```python
from build123d import *

# Parameters (mm, degrees)
SKETCH_1_R             = 10.5
EXTRUDE_1_DEPTH        = 4
SKETCH_4_R             = 2.1
CUT_EXTRUDE_1346_DEPTH = 150.081575092


with BuildPart() as part:
    # 草图1 → 凸台-拉伸1 (new body)
    with BuildSketch(Plane(origin=(0, 0, 0), x_dir=(1, 0, 0), z_dir=(0, 1, 0))):
        with BuildLine():
            Line((0, 0), (60, 0))
            Line((60, 0), (60, 10))
            Line((60, 10), (55.411884484, 19.839245477))
            ThreePointArc((55.411884484, 19.839245477), (55.227167567, 21.861337052), (56.372632354, 23.537906496))
            ThreePointArc((56.372632354, 23.537906496), (70.783850417, 79.017821778), (19.020417199, 103.639990393))
            ThreePointArc((19.020417199, 103.639990393), (16.99979992, 103.840191523), (15.569521651, 105.281468301))
            Line((15.569521651, 105.281468301), (9.668235965, 117.936816295))
            ThreePointArc((9.668235965, 117.936816295), (-13.775496492, 127.647528231), (-25.492512153, 105.139350566))
            Line((-25.492512153, 105.139350566), (0, 10))
            Line((0, 10), (0, 0))
        make_face()
        with Locations(Location((-7.352321507, 110, 0), (0, 0, 270))):
            Circle(SKETCH_1_R, mode=Mode.SUBTRACT)
        with BuildLine():
            Line((26.5, 20.5), (31.5, 20.5))
            ThreePointArc((31.5, 20.5), (32.5, 19.5), (31.5, 18.5))
            Line((31.5, 18.5), (26.5, 18.5))
            ThreePointArc((26.5, 18.5), (25.5, 19.5), (26.5, 20.5))
        make_face(mode=Mode.SUBTRACT)
        with BuildLine():
            Line((-0.975772037, 35.443910191), (2.27680142, 31.646441837))
            ThreePointArc((2.27680142, 31.646441837), (2.167822441, 30.236433474), (0.757814079, 30.345412454))
            Line((0.757814079, 30.345412454), (-2.494759379, 34.142880808))
            ThreePointArc((-2.494759379, 34.142880808), (-2.3857804, 35.552889171), (-0.975772037, 35.443910191))
        make_face(mode=Mode.SUBTRACT)
        with BuildLine():
            Line((60.975772037, 35.443910191), (57.72319858, 31.646441837))
            ThreePointArc((57.72319858, 31.646441837), (57.832177559, 30.236433474), (59.242185921, 30.345412454))
            Line((59.242185921, 30.345412454), (62.494759379, 34.142880808))
            ThreePointArc((62.494759379, 34.142880808), (62.3857804, 35.552889171), (60.975772037, 35.443910191))
        make_face(mode=Mode.SUBTRACT)
    extrude(amount=EXTRUDE_1_DEPTH)

    # 草图4 → Cut-Extrude 1346 (cut, through all)
    with BuildSketch(Plane.XZ):
        with Locations(Location((37, -5, 0), (0, 0, 270))):
            Circle(SKETCH_4_R)
        with Locations(Location((51, -5, 0), (0, 0, 270))):
            Circle(SKETCH_4_R)
        with Locations(Location((9, -5, 0), (0, 0, 90))):
            Circle(SKETCH_4_R)
        with Locations(Location((23, -5, 0), (0, 0, 90))):
            Circle(SKETCH_4_R)
    extrude(amount=-CUT_EXTRUDE_1346_DEPTH, mode=Mode.SUBTRACT)


solid = part.part
```
Model file for the job. Use its own axes, mm. A direction names the side the tool comes from. Give positions to 0.01 mm unless a question says otherwise; leave off trailing zeros. Write each loop counter-clockwise with the first axis right and the second up, starting at its lowest first coordinate (ties: lowest second). Pieces come first, ordered by that corner, then holes. Notation, with made-up numbers: M -21.75,16.5 L 10.25,16.5 A5 cw 10.25,20.5 Z; hole C 59,88 d10. An arc over 180 degrees is marked long. Use a Markdown table: item, result.
1) Cut at A-A (z = -5). List the corners of the cut face in (x, y), and give its area (3 significant figures).
Responses:
| item | result |
|---|---|
| outline | M 0,0 L 6.9,0 L 6.9,4 L 0,4 Z; M 11.1,0 L 20.9,0 L 20.9,4 L 11.1,4 Z; M 25.1,0 L 34.9,0 L 34.9,4 L 25.1,4 Z; M 39.1,0 L 48.9,0 L 48.9,4 L 39.1,4 Z; M 53.1,0 L 60,0 L 60,4 L 53.1,4 Z |
| area | 173 mm2 |
2) Cut at C-C (z = -110). List the corners of the cut face in (x, y).
Responses:
| item | result |
|---|---|
| outline | M -26.13,0 L -17.85,0 L -17.85,4 L -26.13,4 Z; M 3.15,0 L 13.37,0 L 13.37,4 L 3.15,4 Z |
3) Pull direction X, two halves, no side cores. Call faces 1 (the flat face through (24, 0, -65)), 2 (the cylindrical face through (34.95, 1.97, -4.54)), 3 (the cylindrical face through (-13.408, 1.972, -127.777)): +X half, -X half, draft (parallel to the pull), parting line (faces both ways), or undercut.
Responses:
| item | result |
|---|---|
| face 1 | draft |
| face 2 | undercut |
| face 3 | parting line |
4) Pin check, flat tips, straight feed: pin 1 (1.2 mm diameter, centred on y = 1.5, z = -7, fed in from +X); pin 2 (1.2 mm diameter, centred on y = 2, z = -7, fed in from -X); pin 3 (1.5 mm diameter, centred on x = 20.5, y = 2.5, fed in from -Z). Stop position of each tip, or through.
Responses:
| item | result |
|---|---|
| pin 1 | stops at x = 60 |
| pin 2 | stops at x = 0 |
| pin 3 | stops at z = -104.14 |
5) Tool access for faces 4 (the flat face through (59.37, 1.97, -33.57)), 5 (the flat face through (60, 2, -5)), 6 (the flat face through (57.74, 1.97, -14.85)), 7 (the flat face through (0, 2, -5)): list every direction of +Z, -Z, +X, -X, +Y, -Y with a clear straight run to the whole face (end or side of a thin tool).
Responses:
| item | result |
|---|---|
| face 4 | +Y, -Y |
| face 5 | +Z, +X, +Y, -Y |
| face 6 | +X, +Y, -Y |
| face 7 | +Z, -X, +Y, -Y |
6) Drill centre lines: line 1 (X direction, y = 2.6, z = -5); line 2 (Z direction, x = 1, y = 1.7); line 3 (Z direction, x = 57, y = 0.3). Where is each one in solid material? Low to high. Write a range as from..to.
Responses:
| item | result |
|---|---|
| line 1 | x = 0..6.9, 11.1..20.9, 25.1..34.9, 39.1..48.9, 53.1..60 |
| line 2 | z = -126.82..-116.36, -103.64..-33.14, -30.14..0 |
| line 3 | z = -96..-24, -16.43..0 |
7) Cut at B-B (x = -13). List the corners of the cut face in (y, z), and give its area (3 significant figures).
Responses:
| item | result |
|---|---|
| outline | M 0,-127.91 L 4,-127.91 L 4,-118.85 L 0,-118.85 Z; M 0,-101.15 L 4,-101.15 L 4,-58.52 L 0,-58.52 Z |
| area | 207 mm2 |
8) Cut at D-D (y = 1.1). Give the number of separate pieces and of enclosed holes in the cut face, and give its area (3 significant figures).
Responses:
| item | result |
|---|---|
| separate pieces | 1 |
| enclosed holes | 8 |
| area | 8,370 mm2 |
